For this review, use the dimensioned drawing (mm, ordinates from the lowest corner) and the shaded views. A direction names the side the tool comes from. Coordinates: 2 decimals unless noted, no trailing zeros. Write each loop counter-clockwise with the first axis right and the second up, starting at its lowest first coordinate (ties: lowest second). Pieces come first, ordered by that corner, then holes. Notation, with made-up numbers: (30, 37.5) - (77, 37.5) arc R33 cw to (77, 76.5) - close; hole circle Ø6 at (58.25, 54.5). An arc over 180 degrees is marked (long way). One line per item, written item: value.
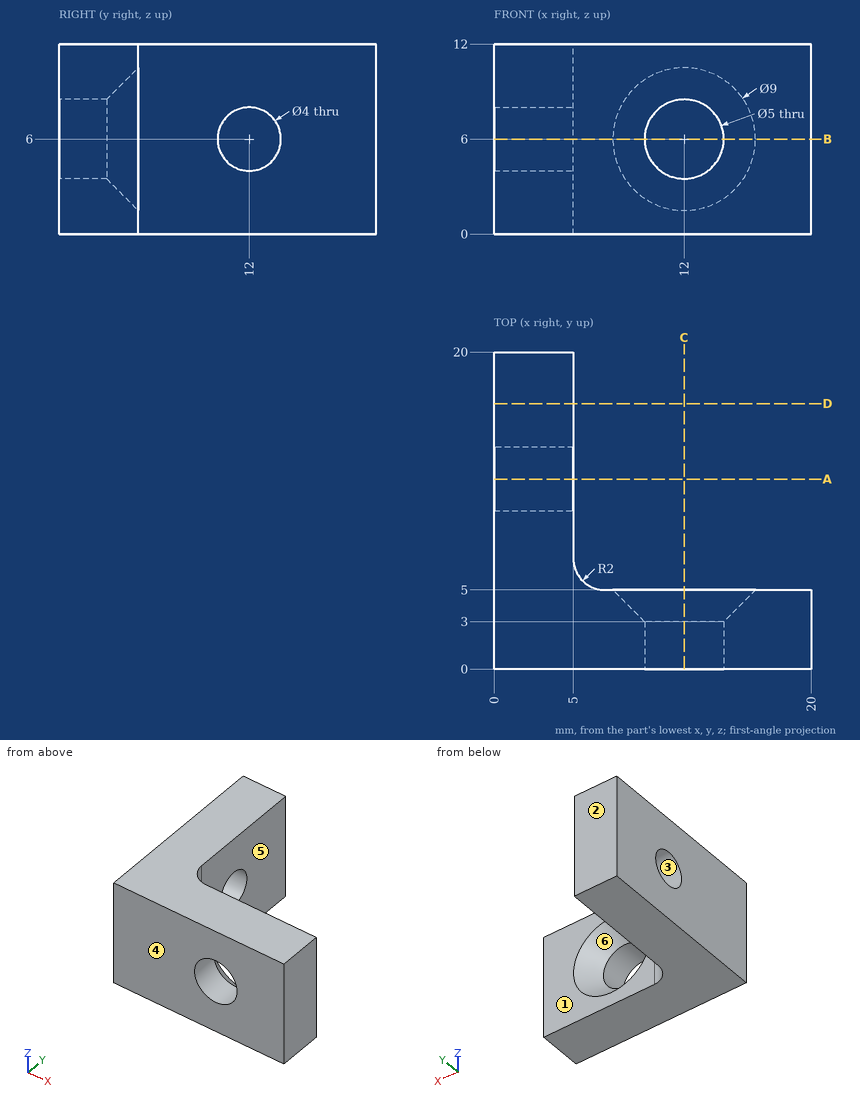
1. For the marked faces 1 and 2, list the 3-axis set-ups (+Z, -Z, +X, -X, +Y, -Y) from which the entire face can be reached by the end or side of a thin tool; tool diameter is ignored.
Answer block:
face 1: +Z, -Z, +X, +Y
face 2: +Z, -Z, +X, -X, +Y
2. Consider section D-D, the plane y = 16.75. Write out the cut boundary in (x, z).
Answer block:
outline: (0, 0) - (5, 0) - (5, 12) - (0, 12) - close
3. Consider section C-C, the plane x = 12. Write out the cut boundary in (y, z).
Answer block:
outline: (0, 0) - (5, 0) - (5, 1.5) - (3, 3.5) - (0, 3.5) - close; (0, 8.5) - (3, 8.5) - (5, 10.5) - (5, 12) - (0, 12) - close
4. Mouldability with a two-part tool opening along Y and no side actions: class the marked faces 3, 4, 5 and 6 as released by +Y, released by -Y, zero draft, split by the parting line, or undercut.
Answer block:
face 3: undercut
face 4: released by -Y
face 5: zero draft
face 6: released by +Y
5. Wall thickness on line 1 along Z through (x, y) = (2.2, 12); line 2 along Z through (x, y) = (12, 2.25); line 3 along X through (y, z) = (1.25, 6): over which ranges is each line inside the solid? List them lowest first.
Answer block:
line 1: z = 0 to 4, 8 to 12
line 2: z = 0 to 3.5, 8.5 to 12
line 3: x = 0 to 9.5, 14.5 to 20
6. Consider section A-A, the plane y = 12. Write out the cut boundary in (x, z), then the cut area to 3 significant figures.
Answer block:
outline: (0, 0) - (5, 0) - (5, 4) - (0, 4) - close; (0, 8) - (5, 8) - (5, 12) - (0, 12) - close
area: 40.0 mm^2
7. Insertion check: pin 1 Ø6 at (y, z) = (10.5, 10.5) entering from +X; pin 2 Ø3.5 at (x, z) = (15, 6) entering from +Y. Each pin has a flat end and moves straight along its axis. Give the tip position at first contact, or say it passes through.
Answer block:
pin 1: stops at x = 5
pin 2: stops at y = 5
8. Consider section B-B, the plane z = 6. Write out the cut boundary in (x, y).
Answer block:
outline: (0, 0) - (9.5, 0) - (9.5, 3) - (7.5, 5) - (7, 5) arc R2 cw to (5, 7) - (5, 10) - (0, 10) - close; (0, 14) - (5, 14) - (5, 20) - (0, 20) - close; (14.5, 0) - (20, 0) - (20, 5) - (16.5, 5) - (14.5, 3) - close
